Geometry: see drawing. Coordinates: mm, zero at the bounding-box minimum. A direction names the side the tool comes from. Coordinates: 2 decimals unless noted, no trailing zeros. Write each loop counter-clockwise with the first axis right and the second up, starting at its lowest first coordinate (ties: lowest second). Pieces come first, ordered by that corner, then holes.
1) Section query D-D (y = 6.75). Output: boundary loops of the cut face in (x, z) (3 decimals).
2) Section query A-A (x = 6.5). Output: boundary loops of the cut face in (y, z).
3) Pin query (flat end, axial travel): pin 1 Ø1.5 at (y, z) = (5.5, 9) entering from +X. Return the tip coordinate at first contact, or that it passes through.
4) Line query: L1, parallel to Z at x = 1.75, y = 2.5; L2, parallel to Z at x = 4, y = 8.75; L3, parallel to X at y = 5.5, z = 12.5. Output: solid intervals per line, ascending.
5) Section query B-B (y = 4.75). Output: boundary loops of the cut face in (x, z).
6) Section query C-C (z = 16). Output: boundary loops of the cut face in (x, y).
7) Set-up query: the marked faces 1, 2 and 3. Return all of +Z, -Z, +X, -X, +Y, -Y with unobstructed straight access to the full face (end or side cutting, diameter ignored); none if empty.
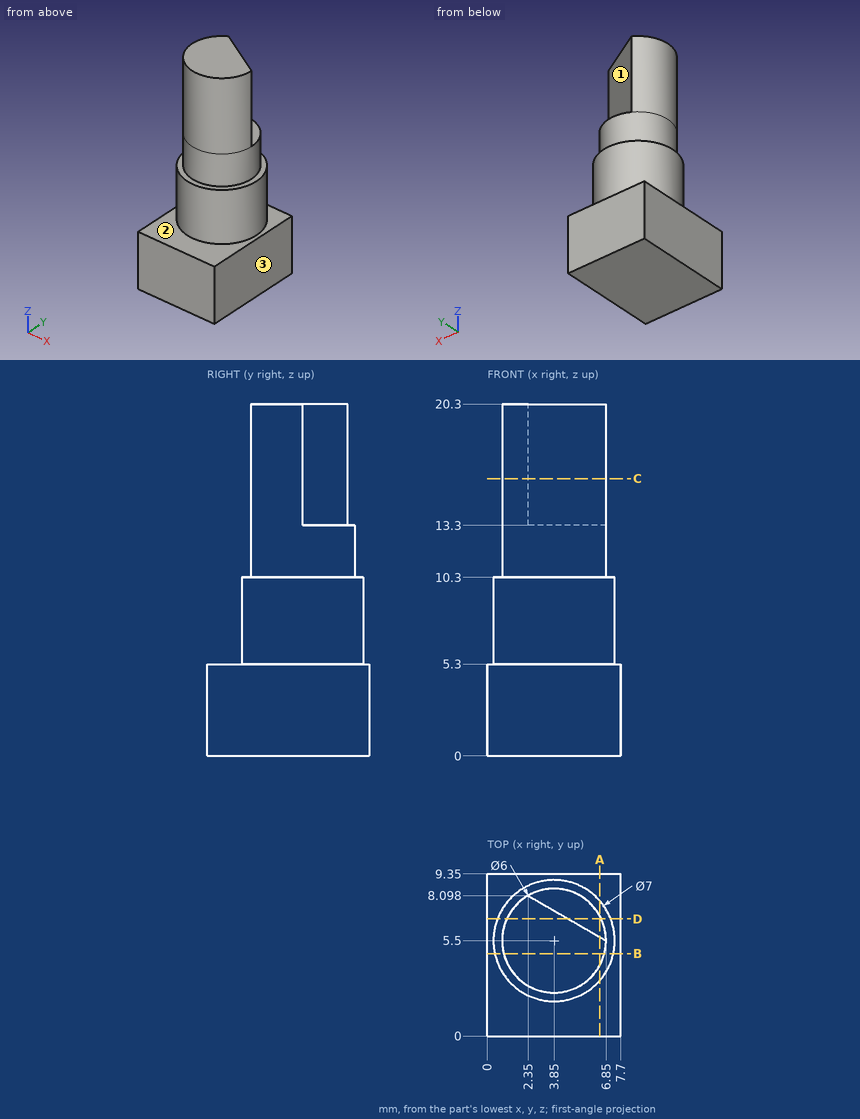
Answer:
1. outline: (0, 0) - (7.7, 0) - (7.7, 5.3) - (7.119, 5.3) - (7.119, 10.3) - (6.577, 10.3) - (6.577, 13.3) - (4.685, 13.3) - (4.685, 20.3) - (1.123, 20.3) - (1.123, 10.3) - (0.581, 10.3) - (0.581, 5.3) - (0, 5.3) - close
2. outline: (0, 0) - (9.35, 0) - (9.35, 5.3) - (7.79, 5.3) - (7.79, 10.3) - (6.91, 10.3) - (6.91, 13.3) - (5.7, 13.3) - (5.7, 20.3) - (4.09, 20.3) - (4.09, 10.3) - (3.21, 10.3) - (3.21, 5.3) - (0, 5.3) - close
3. pin 1: stops at x = 7.35
4. L1: z = 0 to 5.3
4. L2: z = 0 to 10.3
4. L3: x = 0.85 to 6.85
5. outline: (0, 0) - (7.7, 0) - (7.7, 5.3) - (7.27, 5.3) - (7.27, 10.3) - (6.75, 10.3) - (6.75, 20.3) - (0.95, 20.3) - (0.95, 10.3) - (0.43, 10.3) - (0.43, 5.3) - (0, 5.3) - close
6. outline: (2.35, 8.1) arc R3 ccw (long way) to (6.85, 5.5) - close
7. face 1: +Z, +X, +Y
7. face 2: +Z
7. face 3: +Z, -Z, +X, +Y, -Y
